Autodesk Fusion 360 part; units mm, degrees
sketch "Sketch2" plane through (0, 0, 0) normal (0, -1, 0) x (1, 0, 0)
  line L0 (-25, 15) -> (-25, 0)
  line L1 (-25, 0) -> (0, 0)
  line L2 (0, 0) -> (0, 15)
  line L3 (0, 15) -> (-25, 15)
  circle A0 centre (-12.5, 7.5) radius 4.965
  dimension "d7" = 9.93
box "BoxPrimitive2" add length 15 width 25 height 75 placed x (0, 0, 1) y (1, 0, 0) z (0, 1, 0) at (-25, 0, 0) makes body 1
extrude "Extrude1" cut sketch "Sketch2" against normal blind 40 contours A0 bodies 1
box "BoxPrimitive3" add length 30 width 20 height 12.5 placed x (0, -1, 0) y (1, 0, 0) z (0, 0, 1) at (-25, 75, 0) separate body makes body 2
move_body "Move1" bodies 2 to x (1, 0, 0) y (0, 1, 0) z (0, 0, 1) at (2.5, -2.5, 2.5)
combine "Combine1" operation cut target body 1 tool bodies 2
box "BoxPrimitive4" add length 2.5 width 2.5 height 20 placed x (0, 1, 0) y (-1, 0, 0) z (0, 0, 1) at (0, 0, 0) separate body makes body 3
copy_body "CopyPasteBodies1" bodies 3 makes body 4
move_body "Move2" bodies 4 to x (1, 0, 0) y (0, 1, 0) z (0, 0, 1) at (-22.5, 0, 0)
copy_body "CopyPasteBodies2" bodies 3 4 makes body 5 makes body 6
move_body "Move3" bodies 5 6 to x (1, 0, 0) y (0, 1, 0) z (0, 0, 1) at (0, 72.5, 0)
box "BoxPrimitive5" add length 75 width 2.5 height 2.5 placed x (0, 1, 0) y (-1, 0, 0) z (0, 0, 1) at (0, 0, 0) separate body makes body 7
move_body "Move4" bodies 7 to x (1, 0, 0) y (0, 1, 0) z (0, 0, 1) at (0, 0, 17.5)
copy_body "CopyPasteBodies3" bodies 7 makes body 8
move_body "Move5" bodies 8 to x (1, 0, 0) y (0, 1, 0) z (0, 0, 1) at (-22.5, 0, 0)
combine "Combine2" operation add target body 1 tool bodies 6 8 7 3 5 4
Part model, mm, in its own coordinate system. A direction names the side the tool comes from. Give positions to 0.01 mm unless a question says otherwise; leave off trailing zeros. Loops run counter-clockwise (first coordinate to the right, second up) from the corner with the lowest first, then second, coordinate; pieces in that order, holes last. Notation, with made-up numbers: M 23,0.5 L 40,0.5 A21 cw 40,32.5 Z; hole C -20.75,70 d9. An arc over 180 degrees is marked long. Return JSON: item names as keys, results as strings.
1) Saw through at D-D, the plane z = 15.75. List the corners of the cut face in (x, y), then the cut area to 3 significant figures.
Calculated:
{"outline": "M -25,0 L -22.5,0 L -22.5,2.5 L -25,2.5 Z; M -25,72.5 L -22.5,72.5 L -22.5,75 L -25,75 Z; M -2.5,0 L 0,0 L 0,2.5 L -2.5,2.5 Z; M -2.5,72.5 L 0,72.5 L 0,75 L -2.5,75 Z", "area": "25.0 mm2"}
2) Saw through at A-A, the plane y = 10. List the corners of the cut face in (x, z) (3 decimals), then the cut area to 3 significant figures.
Calculated:
{"outline": "M -25,0 L 0,0 L 0,15 L -25,15 Z; M -25,17.5 L -22.5,17.5 L -22.5,20 L -25,20 Z; M -2.5,17.5 L 0,17.5 L 0,20 L -2.5,20 Z; hole C -12.5,7.5 d9.93", "area": "310 mm2"}
3) Saw through at C-C, the plane x = -1.75. List the corners of the cut face in (y, z), then the cut area to 4 significant figures.
Calculated:
{"outline": "M 0,0 L 75,0 L 75,20 L 0,20 Z; hole M 2.5,15 L 72.5,15 L 72.5,17.5 L 2.5,17.5 Z", "area": "1,325 mm2"}
4) 3-axis set-ups, long thin cutter, end or side, ignore diameter. For faces 1 (the face through (-12, 58, 2.5)), 2 (the face through (-2.5, 38, 19)), 3 (the face through (-9.831, 19.72, 11.687)), 4 (the face through (-24, 72.5, 16)): which of +Z, -Z, +X, -X, +Y, -Y reach the whole face in a straight line?
Calculated:
{"face 1": "+Z", "face 2": "+Z, +Y, -Y", "face 3": "-Y", "face 4": "+X, -X"}
5) Flat gauge pins, fed straight in: pin 1 Ø6 at (x, y) = (-16.5, 50.5) entering from +Z; pin 2 Ø0.8 at (x, z) = (-24, 16.5) entering from -Y; pin 3 Ø1 at (x, y) = (-20.5, 19) entering from +Z. Where does each tip first touch, or does it go through?
Calculated:
{"pin 1": "stops at z = 2.5", "pin 2": "stops at y = 0", "pin 3": "stops at z = 15"}
6) Drill centre lines: line 1 (Z direction, x = -1.5, y = 5); line 2 (Y direction, x = -9, z = 10.5); line 3 (Z direction, x = -12.5, y = 16) (3 decimals). Where is each one in solid material? Low to high.
Calculated:
{"line 1": "z = 0 to 15, 17.5 to 20", "line 2": "y = 40 to 42.5, 72.5 to 75", "line 3": "z = 0 to 2.535, 12.465 to 15"}
7) Pull direction X, two halves, no side cores. Call faces 5 (the face through (-22.5, 38, 19)), 6 (the face through (-24, 37, 20)), 7 (the face through (-25, 37, 10)): released by +X, released by -X, zero draft, split by the parting line, or undercut.
Calculated:
{"face 5": "undercut", "face 6": "zero draft", "face 7": "released by -X"}
8) Saw through at B-B, the plane z = 7.5. List the corners of the cut face in (x, y) (3 decimals), then the cut area to 3 significant figures.
Calculated:
{"outline": "M -25,0 L -17.465,0 L -17.465,40 L -7.535,40 L -7.535,0 L 0,0 L 0,75 L -25,75 Z; hole M -22.5,42.5 L -2.5,42.5 L -2.5,72.5 L -22.5,72.5 Z", "area": "878 mm2"}
